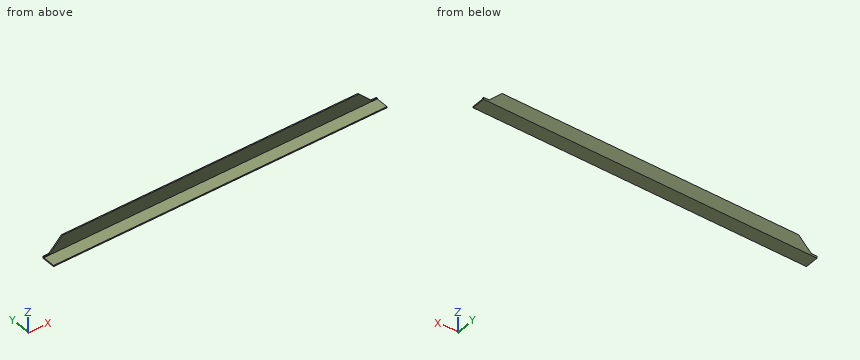
```python
from build123d import *

# Parameters (mm, degrees)
SKETCH_1_W          = 2440
SKETCH_1_H          = 100
EXTRUDE_715_DEPTH   = 8
SKETCH_2_W          = 2440
SKETCH_2_H          = 8
EXTRUDE_1_DEPTH     = 100
CUT_EXTRUDE_1_DEPTH = 1229.846613699


with BuildPart() as part:
    # 草图1 → Extrude 715 (new body)
    with BuildSketch(Plane.XY):
        with Locations((0, 50)):
            Rectangle(SKETCH_1_W, SKETCH_1_H)
    extrude(amount=EXTRUDE_715_DEPTH)

    # 草图2 → 凸台-拉伸1 (add)
    with BuildSketch(Plane.XY.offset(8)):
        with Locations((0, 96)):
            Rectangle(SKETCH_2_W, SKETCH_2_H)
    extrude(amount=EXTRUDE_1_DEPTH)

    # 草图3 → 切除-拉伸1 (cut, through all)
    with BuildSketch(Plane(origin=(0, 100, 0), x_dir=(-1, 0, 0), z_dir=(0, 1, 0))):
        Polygon((-1085, 108), (-1178, 15), (-1220, 15), (-1220, 108), align=None)
        Polygon((1220, 15), (1178, 15), (1085, 108), (1220, 108), align=None)
    extrude(amount=-CUT_EXTRUDE_1_DEPTH, mode=Mode.SUBTRACT)


solid = part.part
```
Design review of the part built by this model. Coordinates are the model's own, in mm. Coordinates: 2 decimals unless noted, no trailing zeros. Order: outer loops, then holes, each group sorted by start corner. A loop starts at its lowest first (then second) coordinate and runs counter-clockwise, first axis right, second up. Notation, with made-up numbers: (6.25, -4.5) - (26.25, -4.5) arc R31 ccw to (26.25, 20.5) - close; hole circle Ø5 at (42.25, 13.5). An arc over 180 degrees is marked (long way). One line per question, with ' | ' between items.
Q1. To check wall thickness, follow line 1 along Y through (x, z) = (-1019.5, 11); line 2 along Z through (x, y) = (-24, 61.5). State the ranges of each line that lie inside material, in increasing order.
Answer key:
line 1: y = 92 to 100 | line 2: z = 0 to 8
Q2. Consider section A-A, the plane x = 552. Give the boundary of the cut face in (y, z).
Answer key:
outline: (0, 0) - (100, 0) - (100, 108) - (92, 108) - (92, 8) - (0, 8) - close
Q3. Consider section B-B, the plane y = 65.5. Give the boundary of the cut face in (x, z), then the cut area to 3 significant figures.
Answer key:
outline: (-1220, 0) - (1220, 0) - (1220, 8) - (-1220, 8) - close | area: 19,500 mm2
Q4. Clearance check with a flat-ended pin moving along its axis: pin 1 Ø6.5 at (x, y) = (1203.5, 94.5) entering from +Z. State where the tip first meets the part, or that it passes through.
Answer key:
pin 1: stops at z = 15
Q5. Consider section C-C, the plane z = 83.5. Give the boundary of the cut face in (x, y).
Answer key:
outline: (-1109.5, 92) - (1109.5, 92) - (1109.5, 100) - (-1109.5, 100) - close
